```python
from build123d import *

# Parameters (mm, degrees)
SKETCH1_R             = 6
BOSS_EXTRUDE1_DEPTH   = 2
SKETCH2_R             = 28.8
BOSS_EXTRUDE2_DEPTH   = 2
SKETCH3_R             = 4
CUT_EXTRUDE1_DEPTH    = 5
M3X0_5_TAPPED_HOLE1_D = 2.5


with BuildPart() as part:
    # Sketch1 → Boss-Extrude1 (new body)
    with BuildSketch(Plane.XY):
        with Locations((0, -108.5)):
            Circle(SKETCH1_R)
    extrude(amount=-BOSS_EXTRUDE1_DEPTH)

    # Sketch2 → Boss-Extrude2 (add)
    with BuildSketch(Plane(origin=(0, 0, -2), x_dir=(-1, 0, 0), z_dir=(0, 0, -1))):
        with Locations((0, -108.5)):
            Circle(SKETCH2_R)
    extrude(amount=BOSS_EXTRUDE2_DEPTH)

    # Sketch3 → Cut-Extrude1 (cut, through all)
    with BuildSketch(Plane.XY):
        with Locations((0, -108.5)):
            Circle(SKETCH3_R)
    extrude(amount=-CUT_EXTRUDE1_DEPTH, mode=Mode.SUBTRACT)

    # M3x0.5 Tapped Hole1 (through all)
    with Locations(Plane.XY.offset(-2)):
        with Locations((-13.435028843, -95.064971157), (13.435028843, -95.064971157), (13.435028843, -121.935028843), (-13.435028843, -121.935028843)):
            Hole(M3X0_5_TAPPED_HOLE1_D / 2)


solid = part.part
```
Could you check a few things on this model? Use its own coordinates, in mm. A direction names the side the tool comes from. Give positions to 0.01 mm unless a question says otherwise; leave off trailing zeros. Write each loop counter-clockwise with the first axis right and the second up, starting at its lowest first coordinate (ties: lowest second). Pieces come first, ordered by that corner, then holes. Notation, with made-up numbers: (-34, -31.5) -> (3, -31.5) arc R28 cw to (3, -3.5) -> close; hole circle Ø5 at (59, -6). An arc over 180 degrees is marked (long way). Write each question's results on one line, items separated by ' | '.
1. I need wall thicknesses on L1, parallel to X at y = -95, z = -2.5; L2, parallel to Y at x = 14, z = -2.3; L3, parallel to Z at x = 17, y = -90.5. Which ranges of each line are inside material? Lowest first, please.
Check sheet entries:
L1: x = -25.44 to -14.68, -12.19 to 12.19, 14.68 to 25.44 | L2: y = -133.67 to -123.05, -120.82 to -96.18, -93.95 to -83.33 | L3: z = -4 to -2
2. I want a section at C-C, the plane x = -13.5. Write out the boundary of the cut face in (y, z), then the cut area to 3 significant figures.
Check sheet entries:
outline: (-133.94, -4) -> (-123.18, -4) -> (-123.18, -2) -> (-133.94, -2) -> close; (-120.69, -4) -> (-96.31, -4) -> (-96.31, -2) -> (-120.69, -2) -> close; (-93.82, -4) -> (-83.06, -4) -> (-83.06, -2) -> (-93.82, -2) -> close | area: 91.8 mm²
3. Will these pins go through, and if not, where does the flat tip stop? pin 1 Ø8 at (x, y) = (5, -97.5) entering from +Z; pin 2 Ø10.5 at (x, y) = (0, -108.5) entering from +Z; pin 3 Ø1.5 at (x, z) = (-21, -1.5) entering from +Y.
Check sheet entries:
pin 1: stops at z = -2 | pin 2: stops at z = 0 | pin 3: stops at y = -88.21
4. I want a section at B-B, the plane x = 0. Write out the boundary of the cut face in (y, z), then the cut area to 3 significant figures.
Check sheet entries:
outline: (-137.3, -4) -> (-112.5, -4) -> (-112.5, 0) -> (-114.5, 0) -> (-114.5, -2) -> (-137.3, -2) -> close; (-104.5, -4) -> (-79.7, -4) -> (-79.7, -2) -> (-102.5, -2) -> (-102.5, 0) -> (-104.5, 0) -> close | area: 107 mm²
5. On a 3-axis mill with a long thin cutter (end or side, diameter ignored), from which of +Z, -Z, +X, -X, +Y, -Y can I reach the whole of each face in a straight line? I mean faces 1 (the flat face through (7, -108, -2)), 2 (the cylindrical face through (12.763, -120.881, -3.014)). Say none if no direction works.
Check sheet entries:
face 1: +Z | face 2: +Z, -Z
6. I want a section at D-D, the plane z = -3.4. Write out the boundary of the cut face in (x, y), then the cut area to 3 significant figures.
Check sheet entries:
outline: circle Ø57.6 at (0, -108.5); hole circle Ø2.5 at (-13.44, -121.94); hole circle Ø2.5 at (-13.44, -95.06); hole circle Ø8 at (0, -108.5); hole circle Ø2.5 at (13.44, -121.94); hole circle Ø2.5 at (13.44, -95.06) | area: 2,540 mm²
7. I want a section at A-A, the plane y = -108.5. Write out the boundary of the cut face in (x, z).
Check sheet entries:
outline: (-28.8, -4) -> (-4, -4) -> (-4, 0) -> (-6, 0) -> (-6, -2) -> (-28.8, -2) -> close; (4, -4) -> (28.8, -4) -> (28.8, -2) -> (6, -2) -> (6, 0) -> (4, 0) -> close
